from build123d import *
from OCP.BRepFilletAPI import BRepFilletAPI_MakeChamfer

# Parameters (mm, degrees)
SKETCH1_W             = 54
SKETCH1_H             = 54
BOSS_EXTRUDE1_DEPTH   = 24
M24_CLEARANCE_HOLE1_D = 26.26
CHAMFER2_SIZE         = 1.8
CHAMFER2_SIZE2        = 0.482308546


with BuildPart() as part:
    # Sketch1 → Boss-Extrude1 (new body)
    with BuildSketch(Plane(origin=(0, 0, 0), x_dir=(1, 0, 0), z_dir=(0, 1, 0))):
        Rectangle(SKETCH1_W, SKETCH1_H)
    extrude(amount=BOSS_EXTRUDE1_DEPTH)

    # Chamfer1
    # the kernel refuses this chamfer: 2, 0.535898385 mm, written as the material it takes off along each edge
    with BuildSketch(Plane(origin=(26.64273441, 22.666666667, -26.154700538), x_dir=(0.25881904510252285, 0, 0.9659258262890678), z_dir=(0.9636113749942796, 0.0691841839943633, -0.2581988897471632)), Plane(origin=(-26.154700538, 22.666666667, -26.64273441), x_dir=(0.9659258262890678, 0, -0.25881904510252285), z_dir=(-0.2581988897471632, 0.0691841839943633, -0.9636113749942796))) as chamfer1_piece_1:
        Polygon((-0.86273015, 0.668267901), (1.20782221, 0.668267901), (-0.34509206, -1.336535802), align=None)
    extrude(amount=0.720242762, mode=Mode.SUBTRACT)
    with BuildSketch(Plane(origin=(26.64273441, 23.154700538, 25.666666667), x_dir=(0.21132486540518758, -0.5773502691896254, -0.788675134594813), z_dir=(0.9636113749942801, 0.2581988897471616, 0.06918418399436459))) as chamfer1_piece_2:
        Polygon((-1.267949192, -0.545638456), (1.267949192, -0.545638456), (0, 1.091276912), align=None)
    extrude(amount=0.720242762, mode=Mode.SUBTRACT)
    with BuildSketch(Plane(origin=(26.154700538, 0.35726559, -25.666666667), x_dir=(0.25881904510252285, 0, 0.9659258262890678), z_dir=(0.2581988897471617, -0.9636113749942801, -0.06918418399436507)), Plane(origin=(-25.666666667, 0.35726559, -26.154700538), x_dir=(0.9659258262890678, 0, -0.25881904510252285), z_dir=(-0.06918418399436507, -0.9636113749942801, -0.2581988897471617)), Plane(origin=(-26.154700538, 0.35726559, 25.666666667), x_dir=(-0.25881904510252124, 0, -0.9659258262890682), z_dir=(-0.2581988897471617, -0.9636113749942801, 0.0691841839943646))) as chamfer1_piece_3:
        Polygon((-1.20782221, -0.668267901), (0.86273015, -0.668267901), (0.34509206, 1.336535802), align=None)
    extrude(amount=0.720242762, mode=Mode.SUBTRACT)
    with BuildSketch(Plane(origin=(26.154700538, 0.35726559, 25.666666667), x_dir=(0.25881904510252124, 0, -0.9659258262890682), z_dir=(0.2581988897471617, -0.9636113749942801, 0.0691841839943646))) as chamfer1_piece_4:
        Polygon((-1.20782221, 0.668267901), (0.86273015, 0.668267901), (0.34509206, -1.336535802), align=None)
    extrude(amount=0.720242762, mode=Mode.SUBTRACT)
    with BuildSketch(Plane(origin=(-26.64273441, 23.154700538, 25.666666667), x_dir=(-0.21132486540518758, -0.5773502691896254, -0.788675134594813), z_dir=(-0.9636113749942801, 0.2581988897471616, 0.06918418399436459))) as chamfer1_piece_5:
        Polygon((-1.267949192, 0.545638456), (1.267949192, 0.545638456), (0, -1.091276912), align=None)
    extrude(amount=0.720242762, mode=Mode.SUBTRACT)
    with BuildSketch(Plane(origin=(27, 24, -32.19344314), x_dir=(0.009967146577157254, -0.9999503267608395, 0), z_dir=(0, 0, 1)), Plane(origin=(-32.19344314, 24, -27), x_dir=(0, -0.9999503267608395, -0.009967146577157254), z_dir=(1, 0, 0)), Plane(origin=(-27, 24, 32.19344314), x_dir=(-0.009967146577157254, -0.9999503267608395, 0), z_dir=(0, 0, -1))) as chamfer1_piece_6:
        with BuildLine():
            Line((2.077377256, 0), (-0.08281798, -0.555806058))
            Line((-0.08281798, -0.555806058), (-0.122815993, -0.555407372))
            ThreePointArc((-0.122815993, -0.555407372), (-0.042771889, -0.277889444), (-0.039998013, 0.000398686))
            Line((-0.039998013, 0.000398686), (0.000398686, 0.039998013))
            ThreePointArc((0.000398686, 0.039998013), (1.038984126, 0.029645766), (2.077775942, 0.039998013))
            Line((2.077775942, 0.039998013), (2.077377256, 0))
        make_face()
    extrude(amount=64.386886281, mode=Mode.SUBTRACT)
    with BuildSketch(Plane(origin=(27, -5.19344314, -27), x_dir=(-0.9905000388259545, 0, -0.13751244702128856), z_dir=(0, 1, 0)), Plane(origin=(-27, -5.19344314, -27), x_dir=(-0.13751244702128856, 0, 0.9905000388259545), z_dir=(0, 1, 0)), Plane(origin=(-27, -5.19344314, 27), x_dir=(0.9905000388259545, 0, 0.13751244702128856), z_dir=(0, 1, 0))) as chamfer1_piece_7:
        with BuildLine():
            Line((0.561942339, 0), (-0.306159862, 2.054692776))
            Line((-0.306159862, 2.054692776), (-0.345779863, 2.049192278))
            ThreePointArc((-0.345779863, 2.049192278), (-0.182445522, 1.023269524), (-0.039620002, -0.005500498))
            Line((-0.039620002, -0.005500498), (0.005500498, -0.039620002))
            ThreePointArc((0.005500498, -0.039620002), (0.281158594, -0.001350019), (0.567442837, -0.039620002))
            Line((0.567442837, -0.039620002), (0.561942339, 0))
        make_face()
    extrude(amount=34.386886281, mode=Mode.SUBTRACT)
    with BuildSketch(Plane(origin=(27, -5.19344314, 27), x_dir=(-0.9905000388259544, 0, 0.13751244702128942), z_dir=(0, 1, 0))) as chamfer1_piece_8:
        with BuildLine():
            Line((0.561942339, 0), (-0.306159862, -2.054692776))
            Line((-0.306159862, -2.054692776), (-0.345779863, -2.049192278))
            ThreePointArc((-0.345779863, -2.049192278), (-0.182445522, -1.023269524), (-0.039620002, 0.005500498))
            Line((-0.039620002, 0.005500498), (0.005500498, 0.039620002))
            ThreePointArc((0.005500498, 0.039620002), (0.281158594, 0.001350019), (0.567442837, 0.039620002))
            Line((0.567442837, 0.039620002), (0.561942339, 0))
        make_face()
    extrude(amount=34.386886281, mode=Mode.SUBTRACT)
    with BuildSketch(Plane(origin=(-32.19344314, 0, -27), x_dir=(0, 0.9905000388259544, -0.1375124470212898), z_dir=(1, 0, 0)), Plane(origin=(27, 0, -32.19344314), x_dir=(0.13751244702128979, 0.9905000388259542, 0), z_dir=(0, 0, 1)), Plane(origin=(32.19344314, 0, 27), x_dir=(0, 0.9905000388259544, 0.1375124470212898), z_dir=(-1, 0, 0)), Plane(origin=(-27, 0, 32.19344314), x_dir=(-0.13751244702128979, 0.9905000388259542, 0), z_dir=(0, 0, -1))) as chamfer1_piece_9:
        with BuildLine():
            Line((0.561942339, 0), (-0.306159862, 2.054692776))
            Line((-0.306159862, 2.054692776), (-0.345779863, 2.049192278))
            ThreePointArc((-0.345779863, 2.049192278), (-0.182445522, 1.023269524), (-0.039620002, -0.005500498))
            Line((-0.039620002, -0.005500498), (0.005500498, -0.039620002))
            ThreePointArc((0.005500498, -0.039620002), (0.281158594, -0.001350019), (0.567442837, -0.039620002))
            Line((0.567442837, -0.039620002), (0.561942339, 0))
        make_face()
    extrude(amount=64.386886281, mode=Mode.SUBTRACT)
    with BuildSketch(Plane(origin=(32.19344314, 24, 27), x_dir=(0, -0.9905000388259544, 0.13751244702128942), z_dir=(-1, 0, 0))) as chamfer1_piece_10:
        with BuildLine():
            Line((0.561942339, 0), (-0.306159862, -2.054692776))
            Line((-0.306159862, -2.054692776), (-0.345779863, -2.049192278))
            ThreePointArc((-0.345779863, -2.049192278), (-0.182445522, -1.023269524), (-0.039620002, 0.005500498))
            Line((-0.039620002, 0.005500498), (0.005500498, 0.039620002))
            ThreePointArc((0.005500498, 0.039620002), (0.281158594, 0.001350019), (0.567442837, 0.039620002))
            Line((0.567442837, 0.039620002), (0.561942339, 0))
        make_face()
    extrude(amount=64.386886281, mode=Mode.SUBTRACT)

    # M24 Clearance Hole1 (through all)
    with Locations(Plane(origin=(0, 24, 0), x_dir=(1, 0, 0), z_dir=(0, 1, 0))):
        with Locations((0, 0)):
            Hole(M24_CLEARANCE_HOLE1_D / 2)

    # Chamfer2: one chamfer whose edges measure the first distance from different faces: ONE call of the kernel's chamfer builder (chamfer() names one face for all edges)
    chamfer2_edges_1 = [part.edges().sort_by_distance(p)[0] for p in [
        (13.13, 24, 0),
    ]]
    chamfer2_side_1 = [part.faces().sort_by_distance(p)[0] for p in [
        (0, 24, -25.725863953),
    ]]
    chamfer2_edges_2 = [part.edges().sort_by_distance(p)[0] for p in [
        (13.13, 0, 0),
    ]]
    chamfer2_side_2 = [part.faces().sort_by_distance(p)[0] for p in [
        (13.13, 12, 0),
    ]]
    chamfer2 = BRepFilletAPI_MakeChamfer(part.part.solid().wrapped)
    for e in chamfer2_edges_1:
        chamfer2.Add(CHAMFER2_SIZE, CHAMFER2_SIZE2, e.wrapped, chamfer2_side_1[0].wrapped)  # the first distance lies on this face
    for e in chamfer2_edges_2:
        chamfer2.Add(CHAMFER2_SIZE, CHAMFER2_SIZE2, e.wrapped, chamfer2_side_2[0].wrapped)  # the first distance lies on this face
    add(Compound.cast(chamfer2.Shape()), mode=Mode.REPLACE)


solid = part.part
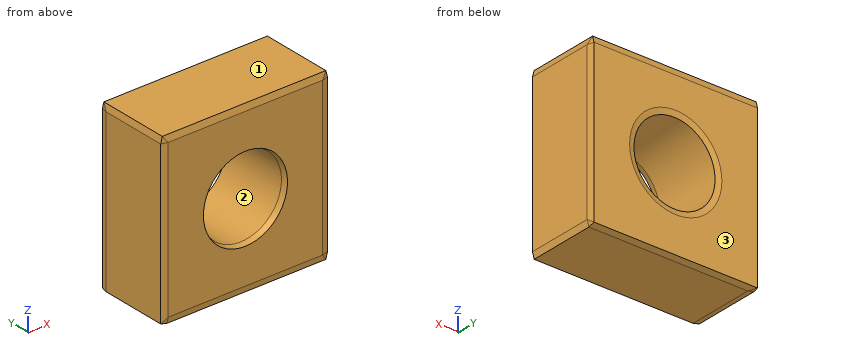
Source: CAD feature listing. Evaluate the final solid. Frame: model axes, mm. Face numbers are marked on the shaded views. Round coordinates to 2 decimals unless told otherwise and drop trailing zeros. Loops run counter-clockwise (first coordinate to the right, second up) from the corner with the lowest first, then second, coordinate; pieces in that order, holes last. Notation, with made-up numbers: M 80.5,-40 L 136.5,-40 A19 cw 136.5,-14 Z; hole C 5,68 d6. An arc over 180 degrees is marked long. Return JSON: item names as keys, results as strings. Group by question number.
1. Section query A-A on z = 0. Output: boundary loops of the cut face in (x, y), and give its area (3 significant figures).
2. Pin query (flat end, axial travel): pin 1 (4 mm diameter, centred on x = -6.5, z = -10.5, fed in from +Y); pin 2 (23.5 mm diameter, centred on x = 0, z = 0, fed in from +Y). Return the tip coordinate at first contact, or that it passes through.
3. Section query B-B on x = 0. Output: boundary loops of the cut face in (y, z), and give its area (3 significant figures).
4. Mould query, pull axis Z, two halves, no side actions, for the marked faces 1, 2 and 3. Classes: released by +Z, released by -Z, zero draft, split by the parting line, or undercut.
5. Material intervals for line 1 along Z through (x, y) = (0, 15.5); line 2 along X through (y, z) = (7, 9), sorted ascending. Write a range as from..to.
6. Section query C-C on y = 20.25. Output: boundary loops of the cut face in (x, z).
Checks:
{
 "1": {"outline": "M -27,0.54 L -25,0 L -13.61,0 L -13.13,1.8 L -13.13,23.52 L -14.93,24 L -26.46,24 L -27,22 Z; M 13.13,1.8 L 13.61,0 L 25,0 L 27,0.54 L 27,22 L 26.46,24 L 14.93,24 L 13.13,23.52 Z", "area": "662 mm²"},
 "2": {"pin 1": "stops at y = 23.84", "pin 2": "passes through"},
 "3": {"outline": "M 0,-25 L 0.54,-27 L 22,-27 L 24,-26.46 L 24,-14.93 L 23.52,-13.13 L 1.8,-13.13 L 0,-13.61 Z; M 0,13.61 L 1.8,13.13 L 23.52,13.13 L 24,14.93 L 24,25 L 23.46,27 L 0.54,27 L 0,25 Z", "area": "662 mm²"},
 "4": {"face 1": "released by +Z", "face 2": "undercut", "face 3": "zero draft"},
 "5": {"line 1": "z = -27..-13.13, 13.13..27", "line 2": "x = -27..-9.56, 9.56..27"},
 "6": {"outline": "M -27,-26.46 L -25,-27 L 26.46,-27 L 27,-25 L 27,25 L 26.46,27 L -26.46,27 L -27,25 Z; hole C 0,0 d26.26"}
}
